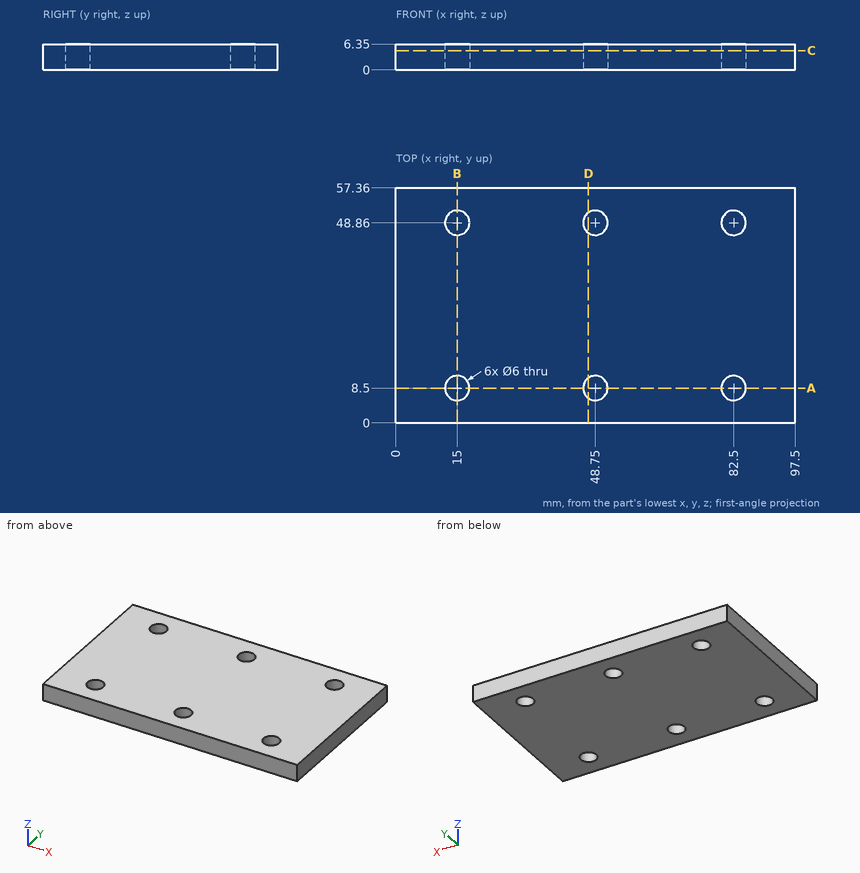
Drawing for the job (mm, zero at the part's lowest x, y, z). Round coordinates to 2 decimals unless told otherwise and drop trailing zeros. Write each loop counter-clockwise with the first axis right and the second up, starting at its lowest first coordinate (ties: lowest second). Pieces come first, ordered by that corner, then holes. Notation, with made-up numbers: M 63,31 L 95,31 A19 ccw 95,42 Z; hole C 74.5,37.25 d9. An arc over 180 degrees is marked long. Answer in a Markdown table with one row per item.
1. Saw through at A-A (y = 8.5). List the corners of the cut face in (x, z), and give its area (3 significant figures).
Geometry check:
| item | result |
|---|---|
| outline | M 0,0 L 12,0 L 12,6.35 L 0,6.35 Z; M 18,0 L 45.75,0 L 45.75,6.35 L 18,6.35 Z; M 51.75,0 L 79.5,0 L 79.5,6.35 L 51.75,6.35 Z; M 85.5,0 L 97.5,0 L 97.5,6.35 L 85.5,6.35 Z |
| area | 505 mm2 |
2. Probe L1, parallel to Y at x = 82.5, z = 1.5; L2, parallel to X at y = 8.5, z = 3; L3, parallel to X at y = 50.5, z = 2. List the from-to ranges inside material, lowest first. Write a range as [from, to].
Geometry check:
| item | result |
|---|---|
| L1 | [0, 5.5], [11.5, 45.86], [51.86, 57.36] |
| L2 | [0, 12], [18, 45.75], [51.75, 79.5], [85.5, 97.5] |
| L3 | [0, 12.49], [17.51, 46.24], [51.26, 79.99], [85.01, 97.5] |
3. Saw through at D-D (x = 47). List the corners of the cut face in (y, z).
Geometry check:
| item | result |
|---|---|
| outline | M 0,0 L 6.06,0 L 6.06,6.35 L 0,6.35 Z; M 10.94,0 L 46.42,0 L 46.42,6.35 L 10.94,6.35 Z; M 51.3,0 L 57.36,0 L 57.36,6.35 L 51.3,6.35 Z |
4. Saw through at C-C (z = 4.75). List the corners of the cut face in (x, y).
Geometry check:
| item | result |
|---|---|
| outline | M 0,0 L 97.5,0 L 97.5,57.36 L 0,57.36 Z; hole C 15,8.5 d6; hole C 15,48.86 d6; hole C 48.75,8.5 d6; hole C 48.75,48.86 d6; hole C 82.5,8.5 d6; hole C 82.5,48.86 d6 |
5. Saw through at B-B (x = 15). List the corners of the cut face in (y, z).
Geometry check:
| item | result |
|---|---|
| outline | M 0,0 L 5.5,0 L 5.5,6.35 L 0,6.35 Z; M 11.5,0 L 45.86,0 L 45.86,6.35 L 11.5,6.35 Z; M 51.86,0 L 57.36,0 L 57.36,6.35 L 51.86,6.35 Z |
6. Flat gauge pin, fed straight in: P1, Ø3, axis at x = 14.5, y = 14.5, coming from the -Z side. Where does the tip first touch, or does it go through?
Geometry check:
| item | result |
|---|---|
| P1 | z = 0 |
